from build123d import *

# Parameters (mm, degrees)
F1_DEPTH   = 6
F4_D       = 2.5
F4_ON_F2_D = 2.5


with BuildPart() as f1:
    # F0 (on Top) → F1 (new body)
    with BuildSketch(Plane.XY):
        Polygon((-16, 0), (0, 0), (0, 8), (-40, 8), (-40, 0), align=None)
        Polygon((31.1769145362, -18), (0, 0), (-16, 0), (27.1769145362, -24.9282032303), align=None)
    extrude(amount=-F1_DEPTH)

    # F4 (through all)
    with Locations(Plane(origin=(0, 0, 0), x_dir=(-0.8660254038, 0.5, 0), z_dir=(0.5, 0.8660254038, 0))):
        with Locations((-33.5, -3), (-2.5, -3)):
            Hole(F4_D / 2)

    # F4 on F2 (through all)
    with Locations(Plane(origin=(0, 8, 0), x_dir=(-1, 0, 0), z_dir=(0, 1, 0))):
        with Locations((6, -3), (36, -3)):
            Hole(F4_ON_F2_D / 2)


solid = f1.part
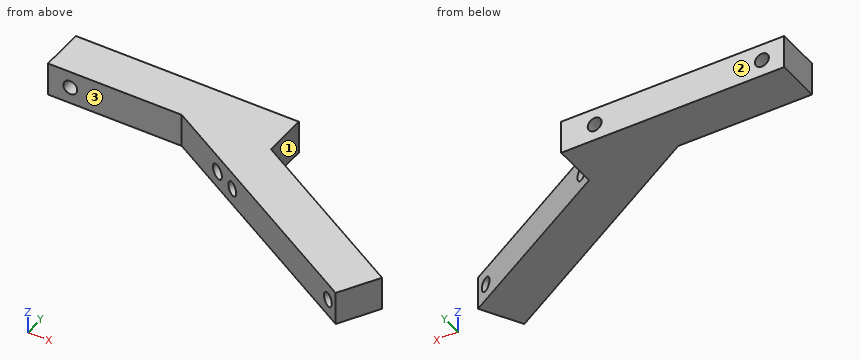
CAD build for the part. Positions are in the model's coordinates, mm. Face numbers are marked on the shaded views. A direction names the side the tool comes from. Round coordinates to 2 decimals unless told otherwise and drop trailing zeros. Write each loop counter-clockwise with the first axis right and the second up, starting at its lowest first coordinate (ties: lowest second). Pieces come first, ordered by that corner, then holes.
(1) 3-axis set-ups, long thin cutter, end or side, ignore diameter. For the marked faces 1, 2 and 3: which of +Z, -Z, +X, -X, +Y, -Y reach the whole face in a straight line?
(2) Probe line 1 along Z through (x, y) = (-36, 3); line 2 along X through (y, z) = (-4, -2.4); line 3 along X through (y, z) = (-20, -2.95). List the from-to ranges inside material, lowest first.
(3) Slice it at D-D, the plane x = -6. Write the cut outline in (y, z), and give its area (3 significant figures).
(4) Drop flat-ended pins along their axis: P1, Ø1.5, axis at y = -13.5, z = -2, coming from the +X side; P2, Ø3, axis at y = 3.5, z = -3, coming from the +X side; P3, Ø2, axis at y = -4.5, z = -4, coming from the +X side; P4, Ø2, axis at x = -36, z = -3, coming from the -Y side. Give the stop position or say it passes through.
(5) Slice it at B-B, the plane z = -3. Write the cut outline in (x, y) (3 decimals), and give its area (3 significant figures).
(6) Slice it at A-A, the plane x = -36. Write the cut outline in (y, z).
(7) Slice it at C-C, the plane y = 2. Write the cut outline in (x, z), and give its area (3 significant figures).
From the geometry:
1. face 1: +Z, -Z, +X, +Y
1. face 2: +Z, -Z, +X, -X, +Y
1. face 3: +Z, -Z, -X, -Y
2. line 1: z = -6 to -4.25, -1.75 to 0
2. line 2: x = -9.07 to -7.1, -4.9 to -0.69, 1.84 to 6.93
2. line 3: x = 18.64 to 25.69, 28.58 to 30.02
3. outline: (-5.77, -6) - (8, -6) - (8, -4.25) - (-5.77, -4.25) - close; (-5.77, -1.75) - (8, -1.75) - (8, 0) - (-5.77, 0) - close
3. area: 48.2 mm2
4. P1: stops at x = 24.68
4. P2: stops at x = 0
4. P3: stops at x = 9.53
4. P4: passes through
5. outline: (-40, 0) - (-37.25, 0) - (-37.25, 8) - (-40, 8) - close; (-34.75, 0) - (-16, 0) - (-7.25, -5.052) - (-7.25, 8) - (-34.75, 8) - close; (-4.75, -6.495) - (-2.917, -7.553) - (1.083, -0.625) - (0, 0) - (0, 8) - (-4.75, 8) - close; (-0.752, -8.803) - (23.929, -23.053) - (27.929, -16.125) - (3.248, -1.875) - close; (26.094, -24.303) - (27.177, -24.928) - (31.177, -18) - (30.094, -17.375) - close
5. area: 569 mm2
6. outline: (0, -6) - (8, -6) - (8, -4.25) - (0, -4.25) - close; (0, -1.75) - (8, -1.75) - (8, 0) - (0, 0) - close
7. outline: (-40, -6) - (0, -6) - (0, 0) - (-40, 0) - close; hole circle Ø2.5 at (-36, -3); hole circle Ø2.5 at (-6, -3)
7. area: 230 mm2
